Answer from the drawing. Dimensions are ordinates in mm from the lowest x, y and z of the part. Coordinates: 2 decimals unless noted, no trailing zeros. Write each loop counter-clockwise with the first axis right and the second up, starting at its lowest first coordinate (ties: lowest second). Pieces come first, ordered by that corner, then holes. Notation, with made-up numbers: (-22, 63.5) -> (24, 63.5) arc R37 cw to (24, 101.5) -> close; hole circle Ø6 at (79.5, 48). An arc over 180 degrees is marked (long way). Answer as a JSON object with one key per item and string values. Group by question number.
(1) Find section C-C (y = 16). Give the vertices of the cut face in (x, z).
(2) Straight lines are drawn through the part: L1, parallel to Y at x = 40, z = 5; L2, parallel to X at y = 43, z = 2.5; L3, parallel to X at y = 5, z = 3. For each, find the intervals that lie inside material, in ascending order.
(3) Find section D-D (x = 35.5). Give the vertices of the cut face in (y, z).
(4) Find section B-B (z = 2.75). Give the vertices of the cut face in (x, y), then the cut area to 3 significant figures.
(5) For a pull along X with two mould halves and no side action, classify the marked faces 1, 2, 3 and 4 as +X half, -X half, draft (parallel to the pull), parting line (faces both ways), or undercut.
(6) Find section A-A (y = 40). Give the vertices of the cut face in (x, z), then the cut area to 3 significant figures.
(7) Flat-ended cylindrical pins translate along their axes: P1, Ø2, axis at y = 16, z = 6.5, coming from the -X side; P2, Ø1.5, axis at x = 51, z = 9.5, coming from the -Y side; P3, Ø3, axis at y = 55, z = 3.5, coming from the +X side. Find the tip coordinate at first contact, or state that the pin passes through.
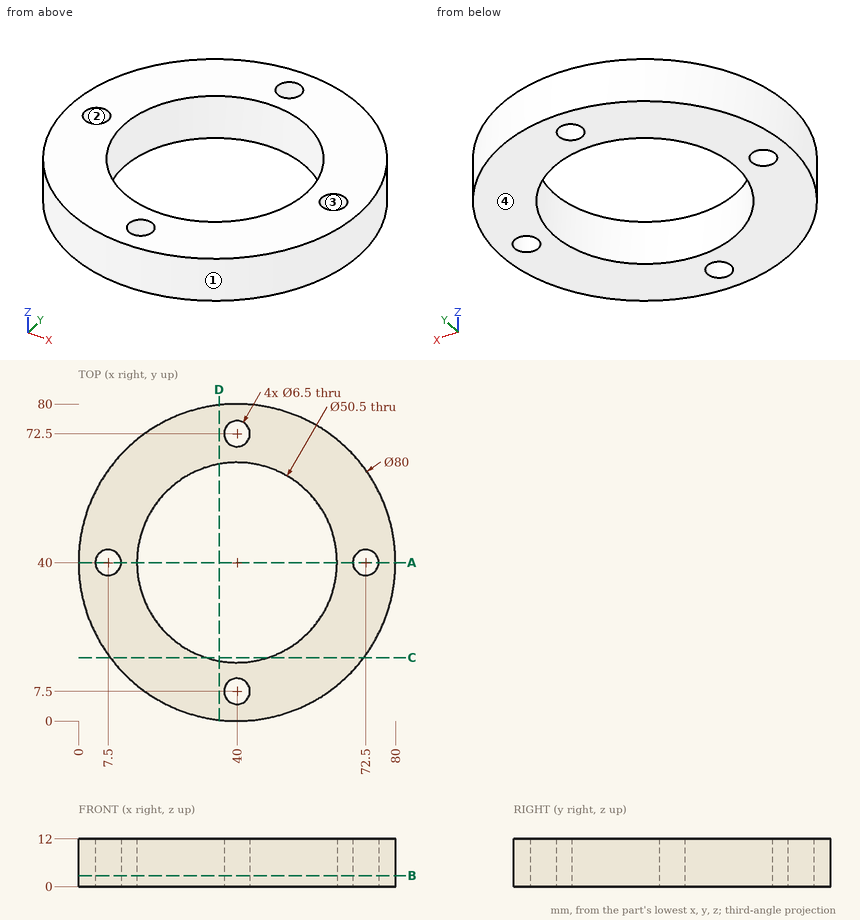
Results below:
{
 "1": {"outline": "(8, 0) -> (32.15, 0) -> (32.15, 12) -> (8, 12) -> close; (47.85, 0) -> (72, 0) -> (72, 12) -> (47.85, 12) -> close"},
 "2": {"L1": "y = 0 to 4.25, 10.75 to 14.75, 65.25 to 69.25, 75.75 to 80", "L2": "x = 0.11 to 6.25, 8.75 to 14.93, 65.07 to 71.25, 73.75 to 79.89", "L3": "x = 20.64 to 37.92, 42.08 to 59.36"},
 "3": {"outline": "(0.25, 0) -> (15.15, 0) -> (15.15, 12) -> (0.25, 12) -> close; (64.85, 0) -> (79.75, 0) -> (79.75, 12) -> (64.85, 12) -> close"},
 "4": {"outline": "circle Ø80 at (40, 40); hole circle Ø6.5 at (7.5, 40); hole circle Ø50.5 at (40, 40); hole circle Ø6.5 at (40, 7.5); hole circle Ø6.5 at (40, 72.5); hole circle Ø6.5 at (72.5, 40)", "area": "2,890 mm2"},
 "5": {"face 1": "parting line", "face 2": "undercut", "face 3": "undercut", "face 4": "draft"},
 "6": {"outline": "(0, 0) -> (4.25, 0) -> (4.25, 12) -> (0, 12) -> close; (10.75, 0) -> (14.75, 0) -> (14.75, 12) -> (10.75, 12) -> close; (65.25, 0) -> (69.25, 0) -> (69.25, 12) -> (65.25, 12) -> close; (75.75, 0) -> (80, 0) -> (80, 12) -> (75.75, 12) -> close", "area": "198 mm2"},
 "7": {"P1": "stops at x = 7.27", "P2": "stops at y = 1.34", "P3": "stops at x = 77.65"}
}
